Geometry: final body of the model. Coordinates: model frame, mm. Face numbers are marked on the shaded views. A direction names the side the tool comes from. Round coordinates to 2 decimals unless told otherwise and drop trailing zeros. Order: outer loops, then holes, each group sorted by start corner. A loop starts at its lowest first (then second) coordinate and runs counter-clockwise, first axis right, second up. Notation, with made-up numbers: M -13,55 L -4,55 A27 ccw -4,72 Z; hole C 20,-38.5 d1. An arc over 180 degrees is marked long. Return JSON: item names as keys, results as strings. Group by question number.
Q1. Access query for the marked faces 1 and 2. Directions: +Z, -Z, +X, -X, +Y, -Y. A direction counts if a zero-diameter tool reaches every point of the face in a straight line with its end or side. Return the directions, or none.
Q2. Ray query, probe 1 along Z at (x, y) = (0.8, 0.2); probe 2 along Z at (x, y) = (0.2, 2.05); probe 3 along X at (y, z) = (-1.15, -1.75). Return the intervals inside material, ascending.
Q3. Contact query for flat-ended pins moving along their axis: pin 1 (0.9 mm diameter, centred on x = -0.5, y = 0.5, fed in from -Z); pin 2 (1.5 mm diameter, centred on x = 0.5, z = 2, fed in from -Y); pin 3 (1.5 mm diameter, centred on x = 0, z = 10.5, fed in from +Y). Output: stop coordinate, or through.
Q4. Mould query, pull axis X, two halves, no side actions, for the marked faces 3, 4 and 5. Classes: released by +X, released by -X, zero draft, split by the parting line, or undercut.
Q5. Cut plane B-B on y = 0. Output: boundary loops of the cut face in (x, z).
Q6. Cut plane C-C on z = 12.75. Output: boundary loops of the cut face in (x, y), and give its area (3 significant figures).
Q7. Cut plane A-A on z = -0.75. Output: boundary loops of the cut face in (x, y), and give its area (3 significant figures).
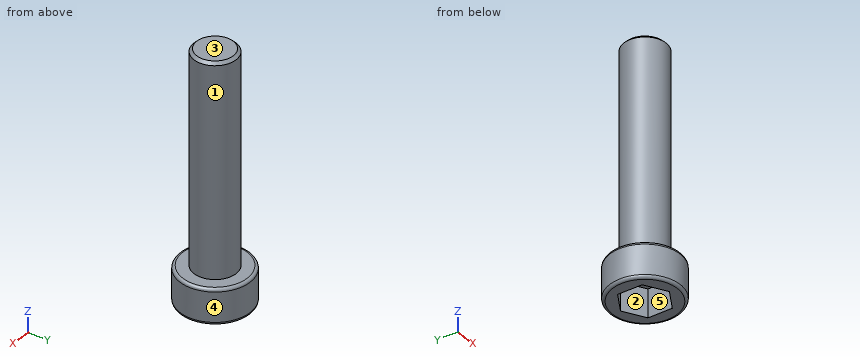
Solid Edge part; units mm, degrees
sketch "Sketch1" plane through (0, 0, 0) normal (0, 0, 1) x (1, 0, 0)
  circle A0 centre (0, 0) radius 1.5
extrude "Protrusion1" add sketch "Sketch1" along normal blind 15
sketch "Sketch2" plane through (0, 0, 0) normal (0, 0, -1) x (0, 1, 0)
  circle A0 centre (0, 0) radius 2.5
extrude "ExtrudedProtrusion_2" add sketch "Sketch2" along normal blind 2.5
fillet "Round_1" radius 0.2 2 edges at (0, -2.5, -2.5) (0, -2.5, 0)
sketch "Sketch3" plane through (0, 0, -2.5) normal (0, 0, -1) x (0, 1, 0)
  line L0 (-0.866, 1.5) -> (-1.7321, 0)
  line L1 (-1.7321, 0) -> (-0.866, -1.5)
  line L2 (-0.866, -1.5) -> (0.866, -1.5)
  line L3 (0.866, -1.5) -> (1.7321, 0)
  line L4 (1.7321, 0) -> (0.866, 1.5)
  line L5 (0.866, 1.5) -> (-0.866, 1.5)
extrude "ExtrudedCutout_1" cut sketch "Sketch3" against normal blind 2
chamfer "Chamfer_1" distance 0.2 angle 45 1 edges at (-1.5, 0, 15) measured on face at (-1.03, -0.97, 15)
cosmetic_thread "Thread1"
Result sheet:
{
 "1": {"face 1": "+Z", "face 2": "-Z"},
 "2": {"probe 1": "z = -0.5 to 15", "probe 2": "z = -2.5 to 0", "probe 3": "x = -2.22 to -1.01, 1.01 to 2.22"},
 "3": {"pin 1": "stops at z = -0.5", "pin 2": "stops at y = -1.5", "pin 3": "stops at y = 1.5"},
 "4": {"face 3": "zero draft", "face 4": "split by the parting line", "face 5": "undercut"},
 "5": {"outline": "M -2.5,-2.3 A0.2 ccw -2.3,-2.5 L -1.5,-2.5 L -1.5,-0.5 L 1.5,-0.5 L 1.5,-2.5 L 2.3,-2.5 A0.2 ccw 2.5,-2.3 L 2.5,-0.2 A0.2 ccw 2.3,0 L 1.5,0 L 1.5,14.8 L 1.3,15 L -1.3,15 L -1.5,14.8 L -1.5,0 L -2.3,0 A0.2 ccw -2.5,-0.2 Z"},
 "6": {"outline": "C 0,0 d3", "area": "7.07 mm²"},
 "7": {"outline": "C 0,0 d5; hole M -1.5,-0.87 L 0,-1.73 L 1.5,-0.87 L 1.5,0.87 L 0,1.73 L -1.5,0.87 Z", "area": "11.8 mm²"}
}
